Could you check a few things on this model? Use its own coordinates, in mm. Face numbers are marked on the shaded views. Give positions to 0.01 mm unless a question says otherwise; leave off trailing zeros. Loops run counter-clockwise (first coordinate to the right, second up) from the corner with the lowest first, then second, coordinate; pieces in that order, holes last. Notation, with made-up numbers: (81, 69) -> (100, 69) arc R30 cw to (100, 95) -> close; hole circle Ø2 at (27.5, 21.25). An arc over 180 degrees is marked (long way). Write item = value, one per line. Start each with the question number.
1) I want a section at A-A (z = -23). List the corners of the cut face in (x, y) for me, and give its area (3 significant figures).
2) I want a section at B-B (x = 2.5). Count the separate pieces of the cut face and the enclosed holes in it, and give its area (3 significant figures).
3) I need wall thicknesses on probe 1 along Z at (x, y) = (2.5, -55.5); probe 2 along Y at (x, z) = (1, -10.5); probe 3 along Y at (x, z) = (1.05, -23.5). Which ranges of each line are inside material? Lowest first, please. Write a range as from..to.
4) I want a section at C-C (y = 9). List the corners of the cut face in (x, z) for me, and give its area (3 significant figures).
5) If we mould it in two halves opening along Y, with no side actions, what happens to the marked faces 1, 2, 3 and 4? For each: +Y half, -Y half, draft (parallel to the pull), parting line (faces both ways), or undercut.
6) I'm going to push a flat-ended pin straight in: pin 1 Ø3 at (x, z) = (2.5, -31.37) entering from +Y. Where does the tip first touch, or does it pass through?
7) I want a section at D-D (z = -13). List the corners of the cut face in (x, y) for me, and give its area (3 significant figures).
from build123d import *

# Parameters (mm, degrees)
SKETCH1_R           = 4.5
BOSS_EXTRUDE1_DEPTH = 5
SKETCH2_R           = 1.4
CUT_EXTRUDE1_DEPTH  = 10


with BuildPart() as part:
    # Sketch1 → Boss-Extrude1 (new body)
    with BuildSketch(Plane(origin=(0, 0, 0), x_dir=(0, 0, -1), z_dir=(1, 0, 0))):
        with BuildLine():
            Line((9.37337158, 19.191374663), (11.37337158, 19.191374663))
            ThreePointArc((11.37337158, 19.191374663), (28.343934329, 12.161937412), (35.37337158, -4.808625337))
            Line((35.37337158, -4.808625337), (35.37337158, -61.308625337))
            Line((35.37337158, -61.308625337), (-14.62662842, -61.308625337))
            Line((-14.62662842, -61.308625337), (-14.62662842, -4.808625337))
            ThreePointArc((-14.62662842, -4.808625337), (-7.597191168, 12.161937412), (9.37337158, 19.191374663))
        make_face()
        with Locations((10.37337158, 1.191374663)):
            Circle(SKETCH1_R, mode=Mode.SUBTRACT)
        with BuildLine():
            Line((-4.55162842, -26.758625337), (-4.55162842, -30.758625337))
            ThreePointArc((-4.55162842, -30.758625337), (-2.67662842, -32.633625337), (-0.80162842, -30.758625337))
            Line((-0.80162842, -30.758625337), (-0.80162842, -26.758625337))
            ThreePointArc((-0.80162842, -26.758625337), (-2.67662842, -24.883625337), (-4.55162842, -26.758625337))
        make_face(mode=Mode.SUBTRACT)
        with BuildLine():
            Line((21.54837158, -26.758625337), (21.54837158, -30.758625337))
            ThreePointArc((21.54837158, -30.758625337), (23.42337158, -32.633625337), (25.29837158, -30.758625337))
            Line((25.29837158, -30.758625337), (25.29837158, -26.758625337))
            ThreePointArc((25.29837158, -26.758625337), (23.42337158, -24.883625337), (21.54837158, -26.758625337))
        make_face(mode=Mode.SUBTRACT)
        with BuildLine():
            Line((25.29837158, -52.858625337), (25.29837158, -56.858625337))
            ThreePointArc((25.29837158, -56.858625337), (23.42337158, -58.733625337), (21.54837158, -56.858625337))
            Line((21.54837158, -56.858625337), (21.54837158, -52.858625337))
            ThreePointArc((21.54837158, -52.858625337), (23.42337158, -50.983625337), (25.29837158, -52.858625337))
        make_face(mode=Mode.SUBTRACT)
        with BuildLine():
            Line((-4.55162842, -52.858625337), (-4.55162842, -56.858625337))
            ThreePointArc((-4.55162842, -56.858625337), (-2.67662842, -58.733625337), (-0.80162842, -56.858625337))
            Line((-0.80162842, -56.858625337), (-0.80162842, -52.858625337))
            ThreePointArc((-0.80162842, -52.858625337), (-2.67662842, -50.983625337), (-4.55162842, -52.858625337))
        make_face(mode=Mode.SUBTRACT)
        with BuildLine():
            Line((-1.12662842, -39.808625337), (-1.12662842, -43.808625337))
            ThreePointArc((-1.12662842, -43.808625337), (10.37337158, -55.308625337), (21.87337158, -43.808625337))
            Line((21.87337158, -43.808625337), (21.87337158, -39.808625337))
            ThreePointArc((21.87337158, -39.808625337), (10.37337158, -28.308625337), (-1.12662842, -39.808625337))
        make_face(mode=Mode.SUBTRACT)
    extrude(amount=BOSS_EXTRUDE1_DEPTH)

    # Sketch2 → Cut-Extrude1 (cut)
    with BuildSketch(Plane(origin=(0, -61.308625337, 0), x_dir=(-1, 0, 0), z_dir=(0, -1, 0))):
        with Locations((-2.5, -10.62662842)):
            Circle(SKETCH2_R)
        with Locations((-2.5, 31.37337158)):
            Circle(SKETCH2_R)
    extrude(amount=-CUT_EXTRUDE1_DEPTH, mode=Mode.SUBTRACT)


solid = part.part
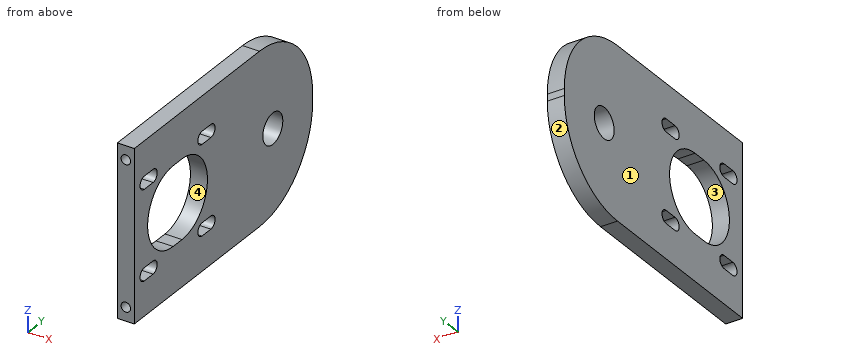
Answer list:
q1.outline = (0, -61.31) -> (5, -61.31) -> (5, -58.69) -> (0, -58.69) -> close; (0, -51.03) -> (5, -51.03) -> (5, -32.59) -> (0, -32.59) -> close; (0, -24.93) -> (5, -24.93) -> (5, 16.19) -> (0, 16.19) -> close
q1.area = 311 mm^2
q2.separate_pieces = 1
q2.enclosed_holes = 6
q2.area = 3,050 mm^2
q3.probe_1 = -35.37..-32.77, -29.97..-25.3, -21.55..0.8, 4.55..9.23, 12.03..14.63
q3.probe_2 = -61.31..-55.31, -28.31..-3.31, 5.69..19.19
q3.probe_3 = -61.31..-58.73, -50.99..-32.63, -24.89..15.9
q4.outline = (0, -31) -> (5, -31) -> (5, 10.26) -> (0, 10.26) -> close
q4.area = 206 mm^2
q5.face_1 = draft
q5.face_2 = +Y half
q5.face_3 = undercut
q5.face_4 = undercut
q6.pin_1 = 10.48
q7.outline = (0, -61.31) -> (5, -61.31) -> (5, -55) -> (0, -55) -> close; (0, -28.61) -> (5, -28.61) -> (5, -2.46) -> (0, -2.46) -> close; (0, 4.85) -> (5, 4.85) -> (5, 19.14) -> (0, 19.14) -> close
q7.area = 234 mm^2
